```python
from build123d import *

# Parameters (mm, degrees)
SKETCH2_W                = 20
SKETCH2_H                = 60
BOSS_EXTRUDE1_DEPTH      = 6.35
SKETCH4_W                = 16.127
SKETCH4_H                = 23.254
CUT_EXTRUDE1_DEPTH       = 64.563531211
M2_CLEARANCE_HOLE1_D     = 2.4
M2_CLEARANCE_HOLE1_DEPTH = 5
M2_CLEARANCE_HOLE1_TIP   = 0.721032743
SKETCH10_W               = 15.127
SKETCH10_H               = 3.175
CUT_EXTRUDE2_DEPTH       = 64.563531211
F_2_CLEARANCE_HOLE1_D    = 2.4384


with BuildPart() as part:
    # Sketch2 → Boss-Extrude1 (new body)
    with BuildSketch(Plane(origin=(0, 0, 0), x_dir=(1, 0, 0), z_dir=(0, 1, 0))):
        with Locations((10, -30)):
            Rectangle(SKETCH2_W, SKETCH2_H)
    extrude(amount=BOSS_EXTRUDE1_DEPTH)

    # Sketch4 → Cut-Extrude1 (cut, through all)
    with BuildSketch(Plane(origin=(0, 6.35, 0), x_dir=(1, 0, 0), z_dir=(0, 1, 0))):
        with Locations((8.0635, -16.5)):
            Rectangle(SKETCH4_W, SKETCH4_H)
    extrude(amount=-CUT_EXTRUDE1_DEPTH, mode=Mode.SUBTRACT)

    # M2 Clearance Hole1
    with Locations(Plane(origin=(0, 6.35, 0), x_dir=(1, 0, 0), z_dir=(0, 1, 0))):
        with Locations((10, -30.5), (10, -2.5)):
            Hole(M2_CLEARANCE_HOLE1_D / 2, depth=M2_CLEARANCE_HOLE1_DEPTH)
            with Locations((0, 0, -(M2_CLEARANCE_HOLE1_DEPTH + M2_CLEARANCE_HOLE1_TIP / 2))):  # 118° drill point
                Cone(0, M2_CLEARANCE_HOLE1_D / 2, M2_CLEARANCE_HOLE1_TIP, mode=Mode.SUBTRACT)

    # Sketch10 → Cut-Extrude2 (cut, through all)
    with BuildSketch(Plane(origin=(20, 0, 0), x_dir=(0, 0, -1), z_dir=(1, 0, 0))):
        with Locations((-52.4365, 4.7625)):
            Rectangle(SKETCH10_W, SKETCH10_H)
    extrude(amount=-CUT_EXTRUDE2_DEPTH, mode=Mode.SUBTRACT)

    # #2 Clearance Hole1 (through all)
    with Locations(Plane(origin=(0, 3.175, 0), x_dir=(1, 0, 0), z_dir=(0, 1, 0))):
        with Locations((10, -48), (4.803847577, -57), (15.196152423, -57)):
            Hole(F_2_CLEARANCE_HOLE1_D / 2)


solid = part.part
```
Can you work these out from the model? Positions are in its coordinate system, mm. A direction names the side the tool comes from. Round coordinates to 2 decimals unless told otherwise and drop trailing zeros. Loops run counter-clockwise (first coordinate to the right, second up) from the corner with the lowest first, then second, coordinate; pieces in that order, holes last.
Item 1: Suppose I cut it at A-A, the plane z = 57. Write out the boundary of the cut face in (x, y) (3 decimals).
Item 2: Will these pins go through, and if not, where does the flat tip stop? pin 1 Ø7.5 at (x, z) = (13, 53) entering from +Y (3 decimals); pin 2 Ø2 at (x, z) = (10, 2.5) entering from +Y; pin 3 Ø1.5 at (x, z) = (10, 48) entering from +Y.
Item 3: If we mould it in two halves opening along Z, with no side actions, what happens to faces 6 (the flat face through (17, 6.35, 27)), 7 (the flat face through (8, 3, 4.873)), 8 (the flat face through (10, 3, 0))? For each: +Z half, -Z half, draft (parallel to the pull), parting line (faces both ways), or undercut.
Item 4: Suppose I cut it at B-B, the plane x = 12.5. Write out the boundary of the cut face in (y, z) (3 decimals), then the cut area to 3 significant figures.
Item 5: Suppose I cut it at C-C, the plane y = 2.25. Write out the boundary of the cut face in (x, z).
Item 6: Suppose I cut it at D-D, the plane x = 14.75. Write out the boundary of the cut face in (y, z) (3 decimals).
Item 7: Please list where these lines run through material, in increasing order: L1, parallel to X at y = 1.9, z = 57; L2, parallel to Z at x = 10, y = 1.85; L3, parallel to Z at x = 10, y = 4.4.
Item 8: Which directions (+Z, -Z, +X, -X, +Y, -Y) give clear straight access to the entire face, cutting with the end or side of a thin tool? Please do faces 1 (the flat face through (8, 3, 28.127)), 2 (the flat face through (20, 3, 30)), 3 (the flat face through (0, 2, 41)), 4 (the cylindrical face through (9.35, 3.81, 29.49)), 5 (the flat face through (10, 5, 44.873)).
Reported:
1. outline: (0, 0) - (3.585, 0) - (3.585, 3.175) - (0, 3.175) - close; (6.023, 0) - (13.977, 0) - (13.977, 3.175) - (6.023, 3.175) - close; (16.415, 0) - (20, 0) - (20, 3.175) - (16.415, 3.175) - close
2. pin 1: stops at y = 3.175
2. pin 2: stops at y = 1.23
2. pin 3: passes through
3. face 6: draft
3. face 7: undercut
3. face 8: -Z half
4. outline: (0, 0) - (6.35, 0) - (6.35, 4.873) - (0, 4.873) - close; (0, 28.127) - (6.35, 28.127) - (6.35, 44.873) - (3.175, 44.873) - (3.175, 60) - (0, 60) - close
4. area: 185 mm2
5. outline: (0, 0) - (20, 0) - (20, 60) - (0, 60) - (0, 28.13) - (16.13, 28.13) - (16.13, 4.87) - (0, 4.87) - close; hole circle Ø2.44 at (4.8, 57); hole circle Ø2.44 at (10, 48); hole circle Ø2.4 at (10, 2.5); hole circle Ø2.4 at (10, 30.5); hole circle Ø2.44 at (15.2, 57)
6. outline: (0, 0) - (6.35, 0) - (6.35, 4.873) - (0, 4.873) - close; (0, 28.127) - (6.35, 28.127) - (6.35, 44.873) - (3.175, 44.873) - (3.175, 55.865) - (0, 55.865) - close; (0, 58.135) - (3.175, 58.135) - (3.175, 60) - (0, 60) - close
7. L1: x = 0 to 3.58, 6.02 to 13.98, 16.42 to 20
7. L2: z = 0 to 1.3, 3.7 to 4.87, 28.13 to 29.3, 31.7 to 46.78, 49.22 to 60
7. L3: z = 0 to 1.3, 3.7 to 4.87, 28.13 to 29.3, 31.7 to 44.87
8. face 1: -X, +Y, -Y
8. face 2: +Z, -Z, +X, +Y, -Y
8. face 3: +Z, -Z, -X, +Y, -Y
8. face 4: +Y
8. face 5: +Z, +X, -X, +Y
